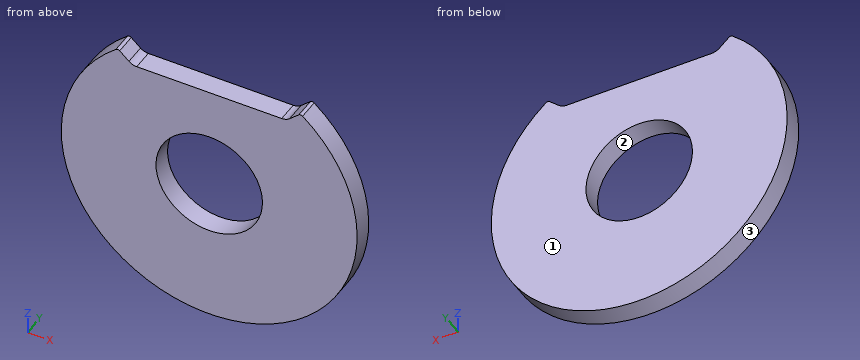
from build123d import *

# Parameters (mm, degrees)
SKETCH1_R           = 18
BOSS_EXTRUDE1_DEPTH = 7


with BuildPart() as part:
    # Sketch1 → Boss-Extrude1 (new body)
    with BuildSketch(Plane(origin=(0, 0, 0), x_dir=(1, 0, 0), z_dir=(0, 1, 0))):
        with BuildLine():
            Line((24.5, -35), (-24.5, -35))
            ThreePointArc((-24.5, -35), (-25.911238902, -35.257219648), (-27.140978616, -35.995797619))
            Line((-27.140978616, -35.995797619), (-30.275171942, -38.751050595))
            ThreePointArc((-30.275171942, -38.751050595), (-30.916482245, -38.999820729), (-31.566751629, -38.775510204))
            ThreePointArc((-31.566751629, -38.775510204), (0, 50), (31.566751629, -38.775510204))
            ThreePointArc((31.566751629, -38.775510204), (30.916482245, -38.999820729), (30.275171942, -38.751050595))
            Line((30.275171942, -38.751050595), (27.140978616, -35.995797619))
            ThreePointArc((27.140978616, -35.995797619), (25.911238902, -35.257219648), (24.5, -35))
        make_face()
        with Locations(Location((0, 0, 0), (0, 0, 270))):
            Circle(SKETCH1_R, mode=Mode.SUBTRACT)
    extrude(amount=BOSS_EXTRUDE1_DEPTH)


solid = part.part
CAD build for the part. Positions are in the model's coordinates, mm. Face numbers are marked on the shaded views. Round coordinates to 2 decimals unless told otherwise and drop trailing zeros. Loops run counter-clockwise (first coordinate to the right, second up) from the corner with the lowest first, then second, coordinate; pieces in that order, holes last. Notation, with made-up numbers: (71.25, -16.75) - (81.25, -16.75) arc R21 ccw to (81.25, 17.25) - close; hole circle Ø4 at (19, 69). An arc over 180 degrees is marked (long way). Put each result on its own line as item: value.
1. Two-plate mould, pull along X, no slides. Class the marked faces 1, 2 and 3: released by +X, released by -X, zero draft, split by the parting line, or undercut.
Geometry check:
face 1: zero draft
face 2: undercut
face 3: split by the parting line
2. Slice it at D-D on x = 44.5. List the corners of the cut face in (y, z).
Geometry check:
outline: (0, -22.8) - (7, -22.8) - (7, 22.8) - (0, 22.8) - close
3. Wall check: line 1 (X direction, y = 4, z = 0); line 2 (Z direction, x = 42, y = 5); line 3 (X direction, y = 3, z = -13.5). Give the ranges that are in metal, low to high.
Geometry check:
line 1: -50 to -18, 18 to 50
line 2: -27.13 to 27.13
line 3: -48.14 to -11.91, 11.91 to 48.14
4. Pin check, flat tips, straight feed: P1, Ø3.5, axis at x = 1, y = 5, coming from the +Z side; P2, Ø6, axis at x = -7, z = -11, coming from the -Y side; P3, Ø4, axis at y = 3.5, z = -32.5, coming from the -X side; P4, Ø1, axis at x = 33.5, y = 5.5, coming from the -Z side. Stop position of each tip, or through.
Geometry check:
P1: z = 35
P2: through
P3: x = -39.62
P4: z = -37.56
5. Slice it at B-B on z = 0. List the corners of the cut face in (x, y).
Geometry check:
outline: (-50, 0) - (-18, 0) - (-18, 7) - (-50, 7) - close; (18, 0) - (50, 0) - (50, 7) - (18, 7) - close
6. Slice it at A-A on x = 0. List the corners of the cut face in (y, z).
Geometry check:
outline: (0, -50) - (7, -50) - (7, -18) - (0, -18) - close; (0, 18) - (7, 18) - (7, 35) - (0, 35) - close
7. Slice it at C-C on y = 5.25. List the corners of the cut face in (x, z).
Geometry check:
outline: (-31.57, 38.78) arc R50 ccw (long way) to (31.57, 38.78) arc R1 ccw to (30.28, 38.75) - (27.14, 36) arc R4 cw to (24.5, 35) - (-24.5, 35) arc R4 cw to (-27.14, 36) - (-30.28, 38.75) arc R1 ccw to start; hole circle Ø36 at (0, 0)
